```python
from build123d import *

# Parameters (mm, degrees)
SKETCH4_R           = 2.5
SKETCH4_R_2         = 1.5
BOSS_EXTRUDE1_DEPTH = 4


with BuildPart() as part:
    # Sketch4 → Boss-Extrude1 (new body)
    with BuildSketch(Plane.XY):
        Polygon((-34.504712973, -20.136303179), (-34.504712973, -76.004712973), (34.504712973, -76.004712973), (34.504712973, -20.136303179), (17.557897552, 21.15), (-17.557897552, 21.15), align=None)
        with Locations((-27.320508076, -27.320508076)):
            Circle(SKETCH4_R, mode=Mode.SUBTRACT)
        with Locations((27.320508076, -27.320508076)):
            Circle(SKETCH4_R, mode=Mode.SUBTRACT)
        with Locations((27.320508076, -68.820508076)):
            Circle(SKETCH4_R, mode=Mode.SUBTRACT)
        with Locations((-27.320508076, -68.820508076)):
            Circle(SKETCH4_R, mode=Mode.SUBTRACT)
        with Locations((-15.5, -15.5)):
            Circle(SKETCH4_R_2, mode=Mode.SUBTRACT)
        with Locations((-15.5, 15.5)):
            Circle(SKETCH4_R_2, mode=Mode.SUBTRACT)
        with Locations((15.5, 15.5)):
            Circle(SKETCH4_R_2, mode=Mode.SUBTRACT)
        with Locations((15.5, -15.5)):
            Circle(SKETCH4_R_2, mode=Mode.SUBTRACT)
        Circle(SKETCH4_R, mode=Mode.SUBTRACT)
    extrude(amount=BOSS_EXTRUDE1_DEPTH)


solid = part.part
```
Input: part model. Units: mm. Frame: model coordinates. Coordinates: 2 decimals unless noted, no trailing zeros. Loops run counter-clockwise (first coordinate to the right, second up) from the corner with the lowest first, then second, coordinate; pieces in that order, holes last. Notation, with made-up numbers: M -23,27.25 L -19,27.25 A35 cw -19,63.25 Z; hole C -3,88 d3. An arc over 180 degrees is marked long. Answer in a Markdown table with one row per item.
1. First-contact query: pin 1 (1.5 mm diameter, centred on x = -25.5, z = 1.5, fed in from +Y). Flat tip, straight axial feed; report the tip coordinate or a pass-through.
Response:
| item | result |
|---|---|
| pin 1 | stops at y = 3.63 |
2. Section D-D, the plane z = 2.5. Count the separate pieces of the cut face and the enclosed holes in it, then the cut area to 3 significant figures.
Response:
| item | result |
|---|---|
| separate pieces | 1 |
| enclosed holes | 9 |
| area | 5,880 mm2 |
3. Section A-A, the plane x = 15.5. Output: boundary loops of the cut face in (y, z), then the cut area to 3 significant figures.
Response:
| item | result |
|---|---|
| outline | M -76,0 L -17,0 L -17,4 L -76,4 Z; M -14,0 L 14,0 L 14,4 L -14,4 Z; M 17,0 L 21.15,0 L 21.15,4 L 17,4 Z |
| area | 365 mm2 |
4. Section B-B, the plane x = 0. Output: boundary loops of the cut face in (y, z), then the cut area to 3 significant figures.
Response:
| item | result |
|---|---|
| outline | M -76,0 L -2.5,0 L -2.5,4 L -76,4 Z; M 2.5,0 L 21.15,0 L 21.15,4 L 2.5,4 Z |
| area | 369 mm2 |
5. Draft query along X for faces 1 (the flat face through (34.505, -48, 2)), 2 (the flat face through (-34.505, -48, 2)), 3 (the flat face through (0, -38, 4)), 4 (the cylindrical face through (14, -15.43, 1.97)). Return one class per face: pulls with the +X half, pulls with the -X half, needs draft (parallel to the pull), parting line crosses it, or undercut.
Response:
| item | result |
|---|---|
| face 1 | pulls with the +X half |
| face 2 | pulls with the -X half |
| face 3 | needs draft |
| face 4 | undercut |
6. Material intervals for line 1 (Y direction, x = -15.5, z = 2.85); line 2 (X direction, y = -29, z = 2.8); line 3 (Y direction, x = 16.5, z = 0.55), sorted ascending.
Response:
| item | result |
|---|---|
| line 1 | y = -76 to -17, -14 to 14, 17 to 21.15 |
| line 2 | x = -34.5 to -29.17, -25.47 to 25.47, 29.17 to 34.5 |
| line 3 | y = -76 to -16.62, -14.38 to 14.38, 16.62 to 21.15 |
7. Section C-C, the plane y = -15.5. Output: boundary loops of the cut face in (x, z), then the cut area to 3 significant figures.
Response:
| item | result |
|---|---|
| outline | M -32.6,0 L -17,0 L -17,4 L -32.6,4 Z; M -14,0 L 14,0 L 14,4 L -14,4 Z; M 17,0 L 32.6,0 L 32.6,4 L 17,4 Z |
| area | 237 mm2 |
